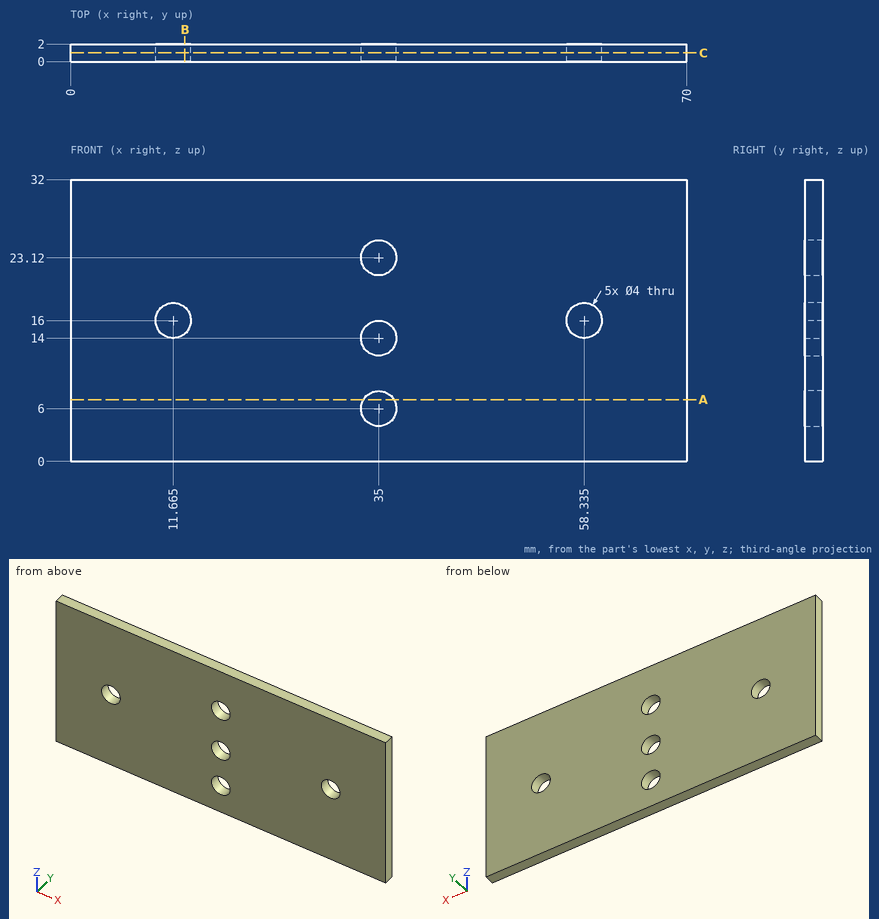
Study the drawing (mm; zero at the part's minimum x, y, z) and answer. Give positions to 0.01 mm unless a question says otherwise; leave off trailing zeros. Order: outer loops, then holes, each group sorted by start corner. A loop starts at its lowest first (then second) coordinate and runs counter-clockwise, first axis right, second up.
1) Find section A-A on z = 7. Write down the section's boundary in (x, y).
Reported:
outline: (0, 0) - (33.27, 0) - (33.27, 2) - (0, 2) - close; (36.73, 0) - (70, 0) - (70, 2) - (36.73, 2) - close
2) Given P1, Ø4, axis at x = 21, z = 8.5, coming from the -Y side, flat-ended and moving along its own axis, determine where the tip first touches the part or whether it passes through.
Reported:
P1: stops at y = 0
3) Find section C-C on y = 1. Write down the section's boundary in (x, z) (3 decimals), then the cut area to 3 significant figures.
Reported:
outline: (0, 0) - (70, 0) - (70, 32) - (0, 32) - close; hole circle Ø4 at (11.665, 16); hole circle Ø4 at (35, 6); hole circle Ø4 at (35, 14); hole circle Ø4 at (35, 23.12); hole circle Ø4 at (58.335, 16)
area: 2,180 mm2
4) Consider line 1 along X through (y, z) = (1.2, 6); line 2 along Z through (x, y) = (58.5, 1.35); line 3 along Z through (x, y) = (34.5, 1.1). Determine where each line is inside the solid, lowest interval first.
Reported:
line 1: x = 0 to 33, 37 to 70
line 2: z = 0 to 14.01, 17.99 to 32
line 3: z = 0 to 4.06, 7.94 to 12.06, 15.94 to 21.18, 25.06 to 32
5) Find section B-B on x = 13. Write down the section's boundary in (y, z).
Reported:
outline: (0, 0) - (2, 0) - (2, 14.51) - (0, 14.51) - close; (0, 17.49) - (2, 17.49) - (2, 32) - (0, 32) - close
